CAD build for the part. Positions are in the model's coordinates, mm. Face numbers are marked on the shaded views. A direction names the side the tool comes from. Give positions to 0.01 mm unless a question says otherwise; leave off trailing zeros. Order: outer loops, then holes, each group sorted by start corner. A loop starts at its lowest first (then second) coordinate and runs counter-clockwise, first axis right, second up. Notation, with made-up numbers: M 8.5,42 L 47.5,42 A32 ccw 47.5,73 Z; hole C -25.75,13.5 d7. An arc over 180 degrees is marked long. Put each result on its own line as item: value. Start each with the question number.
1) Cut at C-C (y = 2). Write the cut outline in (x, z) (3 decimals).
2) Pin check, flat tips, straight feed: pin 1 (0.7 mm diameter, centred on y = 0, z = 1.5, fed in from -X) (3 decimals); pin 2 (0.7 mm diameter, centred on y = -0.5, z = -1.5, fed in from +X) (3 decimals); pin 3 (0.5 mm diameter, centred on x = -2.5, y = 0, fed in from -Z) (3 decimals). Stop position of each tip, or through.
3) Cut at D-D (x = -3). Write the cut outline in (y, z) (3 decimals).
4) Drill centre lines: line 1 (X direction, y = 1.5, z = -0.9); line 2 (Z direction, x = -2.5, y = 9.75) (3 decimals); line 3 (Y direction, x = 0.75, z = -1). Where is each one in solid material? Low to high. Write a range as [from, to].
5) Tool access for the marked faces 1, 2 and 3: list every direction of +Z, -Z, +X, -X, +Y, -Y with a clear straight run to the whole face (end or side of a thin tool).
6) Cut at A-A (y = -0.75). Write the cut outline in (x, z) (3 decimals).
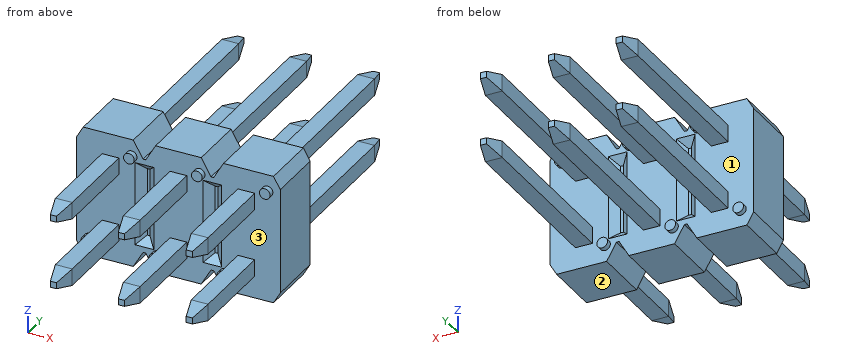
```python
from build123d import *

# Parameters (mm, degrees)
BOSS_EXTRUDE1_DEPTH      = 2.14
BOSS_EXTRUDE2_START      = -2.34
SKETCH2_R                = 0.2
BOSS_EXTRUDE2_DEPTH      = 2.54
LPATTERN1_COUNT          = 3
LPATTERN1_PITCH          = 2.54
SKETCH3_W                = 0.1
SKETCH3_H                = 2.54
CUT_EXTRUDE1_DEPTH       = 0.3
CHAMFER1_SIZE            = 0.3
CHAMFER1_OF_MIRROR2_SIZE = 0.3
SKETCH6_W                = 0.63
SKETCH6_H                = 0.63
CHAMFER2_SIZE            = 0.2
CHAMFER2_SIZE2           = 0.746410162
CHAMFER3_SIZE            = 0.2
CHAMFER3_SIZE2           = 0.746410162
LPATTERN2_START          = -1.585
LPATTERN2_DEPTH          = 0.63
LPATTERN2_START_2        = -1
LPATTERN2_2_DEPTH        = 5
MIRROR4_START            = -2.655
MIRROR4_DEPTH            = 0.23
MIRROR4_START_2          = -0.115
MIRROR4_2_DEPTH          = 0.23
MIRROR4_START_3          = 2.425
MIRROR4_3_DEPTH          = 0.23
MIRROR4_START_4          = 0.955
MIRROR4_4_DEPTH          = 0.63
MIRROR4_START_5          = -4
MIRROR4_5_DEPTH          = 8


with BuildPart() as part:
    # Sketch1 → Boss-Extrude1 (new body)
    with BuildSketch(Plane(origin=(0, 1.36, 0), x_dir=(1, 0, 0), z_dir=(0, 1, 0))):
        Polygon((-1.686617421, 2.415), (-1.32, 1.78), (-1.22, 1.78), (-0.853382579, 2.415), (0.853382579, 2.415), (1.22, 1.78), (1.32, 1.78), (1.686617421, 2.415), (3.556, 2.415), (3.81, 1.975059095), (3.81, -1.975059095), (3.556, -2.415), (1.686617421, -2.415), (1.32, -1.78), (1.22, -1.78), (0.853382579, -2.415), (-0.853382579, -2.415), (-1.22, -1.78), (-1.32, -1.78), (-1.686617421, -2.415), (-3.556, -2.415), (-3.81, -1.975059095), (-3.81, 1.975059095), (-3.556, 2.415), align=None)
    extrude(amount=BOSS_EXTRUDE1_DEPTH)

    # Sketch2 → Boss-Extrude2 (add)
    with BuildSketch(Plane(origin=(0, 3.5, 0), x_dir=(1, 0, 0), z_dir=(0, 1, 0)).offset(BOSS_EXTRUDE2_START)):
        with Locations(Location((-3.3325, 1.785, 0), (0, 0, 270))):
            Circle(SKETCH2_R)
        with Locations(Location((-1.7475, -1.785, 0), (0, 0, 270))):
            Circle(SKETCH2_R)
    boss_extrude2 = extrude(amount=BOSS_EXTRUDE2_DEPTH)

    # LPattern1: Boss-Extrude2 ×3
    with Locations(*[(i * LPATTERN1_PITCH, 0, 0) for i in range(1, LPATTERN1_COUNT)]):
        add(boss_extrude2)

    # Sketch3 → Cut-Extrude1 (cut)
    with BuildSketch(Plane(origin=(0, 3.5, 0), x_dir=(1, 0, 0), z_dir=(0, 1, 0))):
        with Locations((-1.27, 0)):
            Rectangle(SKETCH3_W, SKETCH3_H)
        with Locations((1.27, 0)):
            Rectangle(SKETCH3_W, SKETCH3_H)
    cut_extrude1 = extrude(amount=-CUT_EXTRUDE1_DEPTH, mode=Mode.SUBTRACT)

    # Chamfer1
    chamfer1_edges = [part.edges().sort_by_distance(p)[0] for p in [
        (-1.27, 3.5, 1.27),
        (-1.22, 3.5, 0),
        (-1.27, 3.5, -1.27),
        (-1.32, 3.5, 0),
        (1.27, 3.5, 1.27),
        (1.32, 3.5, 0),
        (1.22, 3.5, 0),
        (1.27, 3.5, -1.27),
    ]]
    chamfer(chamfer1_edges, length=CHAMFER1_SIZE - 0.0001)  # a hair under: the kernel refuses the full size

    # Mirror2: Cut-Extrude1 across plane
    add(cut_extrude1.mirror(Plane.ZX.offset(2.43)), mode=Mode.SUBTRACT)

    # Chamfer1 of Mirror2
    chamfer1_of_mirror2_edges = [part.edges().sort_by_distance(p)[0] for p in [
        (-1.27, 1.36, 1.27),
        (-1.22, 1.36, 0),
        (-1.27, 1.36, -1.27),
        (-1.32, 1.36, 0),
        (1.27, 1.36, 1.27),
        (1.32, 1.36, 0),
        (1.22, 1.36, 0),
        (1.27, 1.36, -1.27),
    ]]
    chamfer(chamfer1_of_mirror2_edges, length=CHAMFER1_OF_MIRROR2_SIZE - 0.0001)  # a hair under: the kernel refuses the full size

    # Sweep1: sweep along a path in Sketch5
    with BuildLine(Plane(origin=(-2.54, 0, 0), x_dir=(0, 0, -1), z_dir=(1, 0, 0))) as sweep1_path:
        Line((1.27, 10.7), (1.27, -2.73))
    # Sketch6 → Sweep1 (sweep)
    with BuildSketch(Plane(origin=(0, 10.7, 0), x_dir=(1, 0, 0), z_dir=(0, 1, 0))):
        with Locations((-2.54, 1.27)):
            Rectangle(SKETCH6_W, SKETCH6_H)
    sweep(path=sweep1_path.line)

    # Chamfer2
    chamfer2_edges = [part.edges().sort_by_distance(p)[0] for p in [
        (-2.225, -2.73, -1.27),
        (-2.54, -2.73, -0.955),
        (-2.855, -2.73, -1.27),
        (-2.54, -2.73, -1.585),
    ]]
    chamfer2_side = [part.faces().sort_by_distance(p)[0] for p in [
        (-2.54, -2.73, -1.27),
    ]]
    chamfer(chamfer2_edges, length=CHAMFER2_SIZE, length2=CHAMFER2_SIZE2, reference=chamfer2_side[0])

    # Chamfer3
    chamfer3_edges = [part.edges().sort_by_distance(p)[0] for p in [
        (-2.225, 10.7, -1.27),
        (-2.54, 10.7, -1.585),
        (-2.855, 10.7, -1.27),
        (-2.54, 10.7, -0.955),
    ]]
    chamfer3_side = [part.faces().sort_by_distance(p)[0] for p in [
        (-2.54, 10.7, -1.27),
    ]]
    chamfer(chamfer3_edges, length=CHAMFER3_SIZE, length2=CHAMFER3_SIZE2, reference=chamfer3_side[0])

    # LPattern2: read off the stored shape, not the designer's step
    # LPattern2 outline → LPattern2 (add)
    with BuildSketch(Plane.XY.offset(LPATTERN2_START)):
        Polygon((2.225, 9.953589838), (2.225, 3.5), (2.855, 3.5), (2.855, 9.953589838), (2.655, 10.7), (2.425, 10.7), align=None)
        Polygon((0.115, 10.7), (-0.115, 10.7), (-0.315, 9.953589838), (-0.315, 3.5), (0.315, 3.5), (0.315, 9.953589838), align=None)
        Polygon((-0.315, -1.983589838), (-0.115, -2.73), (0.115, -2.73), (0.315, -1.983589838), (0.315, 1.36), (-0.315, 1.36), align=None)
        Polygon((2.855, 1.36), (2.225, 1.36), (2.225, -1.983589838), (2.425, -2.73), (2.655, -2.73), (2.855, -1.983589838), align=None)
    extrude(amount=LPATTERN2_DEPTH)

    # LPattern2 2 outline → LPattern2 2 (cut)
    with BuildSketch(Plane.YZ.offset(LPATTERN2_START_2)):
        Polygon((-2.73, -0.955), (-2.73, -1.155), (-1.983589838, -0.955), align=None)
        Polygon((-1.983589838, -1.585), (-2.73, -1.385), (-2.73, -1.585), align=None)
        Polygon((9.953589838, -0.955), (10.7, -1.155), (10.7, -0.955), align=None)
        Polygon((10.7, -1.385), (9.953589838, -1.585), (10.7, -1.585), align=None)
    extrude(amount=LPATTERN2_2_DEPTH, mode=Mode.SUBTRACT)

    # Mirror4: read off the stored shape, not the designer's step
    # Mirror4 outline → Mirror4 (add)
    with BuildSketch(Plane.YZ.offset(MIRROR4_START)):
        Polygon((10.7, 1.155), (10.7, 1.385), (9.953589838, 1.585), (3.5, 1.585), (3.5, 0.955), (9.953589838, 0.955), align=None)
        Polygon((-1.983589838, 1.585), (-2.73, 1.385), (-2.73, 1.155), (-1.983589838, 0.955), (1.36, 0.955), (1.36, 1.585), align=None)
    extrude(amount=MIRROR4_DEPTH)

    # Mirror4 2 outline → Mirror4 2 (add)
    with BuildSketch(Plane.YZ.offset(MIRROR4_START_2)):
        Polygon((10.7, 1.155), (10.7, 1.385), (9.953589838, 1.585), (3.5, 1.585), (3.5, 0.955), (9.953589838, 0.955), align=None)
        Polygon((-1.983589838, 1.585), (-2.73, 1.385), (-2.73, 1.155), (-1.983589838, 0.955), (1.36, 0.955), (1.36, 1.585), align=None)
    extrude(amount=MIRROR4_2_DEPTH)

    # Mirror4 3 outline → Mirror4 3 (add)
    with BuildSketch(Plane.YZ.offset(MIRROR4_START_3)):
        Polygon((10.7, 1.155), (10.7, 1.385), (9.953589838, 1.585), (3.5, 1.585), (3.5, 0.955), (9.953589838, 0.955), align=None)
        Polygon((-1.983589838, 1.585), (-2.73, 1.385), (-2.73, 1.155), (-1.983589838, 0.955), (1.36, 0.955), (1.36, 1.585), align=None)
    extrude(amount=MIRROR4_3_DEPTH)

    # Mirror4 4 outline → Mirror4 4 (add)
    with BuildSketch(Plane.XY.offset(MIRROR4_START_4)):
        Polygon((-2.655, 1.36), (-2.855, 1.36), (-2.855, -1.983589838), (-2.655, -2.73), align=None)
        Polygon((2.855, 1.36), (2.655, 1.36), (2.655, -2.73), (2.855, -1.983589838), align=None)
        Polygon((2.425, 1.36), (2.225, 1.36), (2.225, -1.983589838), (2.425, -2.73), align=None)
        Polygon((0.315, 1.36), (0.115, 1.36), (0.115, -2.73), (0.315, -1.983589838), align=None)
        Polygon((-0.115, 1.36), (-0.315, 1.36), (-0.315, -1.983589838), (-0.115, -2.73), align=None)
        Polygon((-2.225, 1.36), (-2.425, 1.36), (-2.425, -2.73), (-2.225, -1.983589838), align=None)
        Polygon((-2.655, 10.7), (-2.855, 9.953589838), (-2.855, 3.5), (-2.655, 3.5), align=None)
        Polygon((2.655, 10.7), (2.655, 3.5), (2.855, 3.5), (2.855, 9.953589838), align=None)
        Polygon((2.225, 9.953589838), (2.225, 3.5), (2.425, 3.5), (2.425, 10.7), align=None)
        Polygon((0.115, 10.7), (0.115, 3.5), (0.315, 3.5), (0.315, 9.953589838), align=None)
        Polygon((-0.315, 9.953589838), (-0.315, 3.5), (-0.115, 3.5), (-0.115, 10.7), align=None)
        Polygon((-2.425, 10.7), (-2.425, 3.5), (-2.225, 3.5), (-2.225, 9.953589838), align=None)
    extrude(amount=MIRROR4_4_DEPTH)

    # Mirror4 5 outline → Mirror4 5 (cut)
    with BuildSketch(Plane.YZ.offset(MIRROR4_START_5)):
        Polygon((-2.73, 1.155), (-2.73, 0.955), (-1.983589838, 0.955), align=None)
        Polygon((-2.73, 1.585), (-2.73, 1.385), (-1.983589838, 1.585), align=None)
        Polygon((10.7, 1.585), (9.953589838, 1.585), (10.7, 1.385), align=None)
        Polygon((10.7, 1.155), (9.953589838, 0.955), (10.7, 0.955), align=None)
    extrude(amount=MIRROR4_5_DEPTH, mode=Mode.SUBTRACT)


solid = part.part
```
Solution:
1. outline: M -3.81,-1.975 L -3.556,-2.415 L -1.687,-2.415 L -1.32,-1.78 L -1.22,-1.78 L -0.853,-2.415 L 0.853,-2.415 L 1.22,-1.78 L 1.32,-1.78 L 1.687,-2.415 L 3.556,-2.415 L 3.81,-1.975 L 3.81,1.975 L 3.556,2.415 L 1.687,2.415 L 1.32,1.78 L 1.22,1.78 L 0.853,2.415 L -0.853,2.415 L -1.22,1.78 L -1.32,1.78 L -1.687,2.415 L -3.556,2.415 L -3.81,1.975 Z
2. pin 1: x = -2.855
2. pin 2: x = 2.855
2. pin 3: z = -1.585
3. outline: M 1.36,-2.415 L 3.5,-2.415 L 3.5,2.415 L 1.36,2.415 Z
4. line 1: [-3.81, -1.48], [-1.06, 1.06], [1.48, 3.81]
4. line 2: [-1.585, -0.955], [0.955, 1.585]
4. line 3: [1.36, 3.5]
5. face 1: +Y
5. face 2: -Z, +X, -X, +Y, -Y
5. face 3: -Y
6. outline: M -2.855,-1.585 L -2.225,-1.585 L -2.225,-0.955 L -2.855,-0.955 Z; M -2.855,0.955 L -2.225,0.955 L -2.225,1.585 L -2.855,1.585 Z; M -0.315,-1.585 L 0.315,-1.585 L 0.315,-0.955 L -0.315,-0.955 Z; M -0.315,0.955 L 0.315,0.955 L 0.315,1.585 L -0.315,1.585 Z; M 2.225,-1.585 L 2.855,-1.585 L 2.855,-0.955 L 2.225,-0.955 Z; M 2.225,0.955 L 2.855,0.955 L 2.855,1.585 L 2.225,1.585 Z
